```python
from build123d import *

# Parameters (mm, degrees)
F0_R     = 15
F0_R_2   = 10
F1_DEPTH = 25
F2_DEPTH = 50
F3_R     = 3


with BuildPart() as f1:
    # F0 (on Front) → F1 (new body)
    with BuildSketch(Plane.XZ):
        with BuildLine():
            ThreePointArc((-6.25, -29.341736), (18.874586, -23.318448), (30, 0))
            ThreePointArc((30, 0), (18.874586, 23.318448), (-6.25, 29.341736))
            ThreePointArc((-6.25, 29.341736), (-30, 0), (-6.25, -29.341736))
        make_face()
        Circle(F0_R, mode=Mode.SUBTRACT)
        with BuildLine():
            ThreePointArc((-6.25, -29.341736), (-30, 0), (-6.25, 29.341736))
            Line((-6.25, 29.341736), (-63.645833, 17.116013))
            ThreePointArc((-63.645833, 17.116013), (-48.989825, 13.602428), (-42.5, 0))
            ThreePointArc((-42.5, 0), (-48.989825, -13.602428), (-63.645833, -17.116013))
            Line((-63.645833, -17.116013), (-6.25, -29.341736))
        make_face()
        with BuildLine():
            ThreePointArc((-42.5, 0), (-48.989825, 13.602428), (-63.645833, 17.116013))
            ThreePointArc((-63.645833, 17.116013), (-77.5, 0), (-63.645833, -17.116013))
            ThreePointArc((-63.645833, -17.116013), (-48.989825, -13.602428), (-42.5, 0))
        make_face()
        with Locations((-60, 0)):
            Circle(F0_R_2, mode=Mode.SUBTRACT)
    extrude(amount=F1_DEPTH)

    # F0 (on Front) → F2 (join)
    with BuildSketch(Plane.XZ):
        with BuildLine():
            ThreePointArc((-6.25, -29.341736), (18.874586, -23.318448), (30, 0))
            ThreePointArc((30, 0), (18.874586, 23.318448), (-6.25, 29.341736))
            ThreePointArc((-6.25, 29.341736), (-30, 0), (-6.25, -29.341736))
        make_face()
        Circle(F0_R, mode=Mode.SUBTRACT)
    extrude(amount=F2_DEPTH)

    # F3
    f3_edges = [f1.edges().sort_by_distance(p)[0] for p in [
        (6.25, -50, -29.341736),
        (30, 0, 0),
        (-34.947917, 0, -23.228875),
        (-77.5, 0, 0),
        (-34.947917, 0, 23.228875),
    ]]
    fillet(f3_edges, radius=F3_R)


solid = f1.part
```
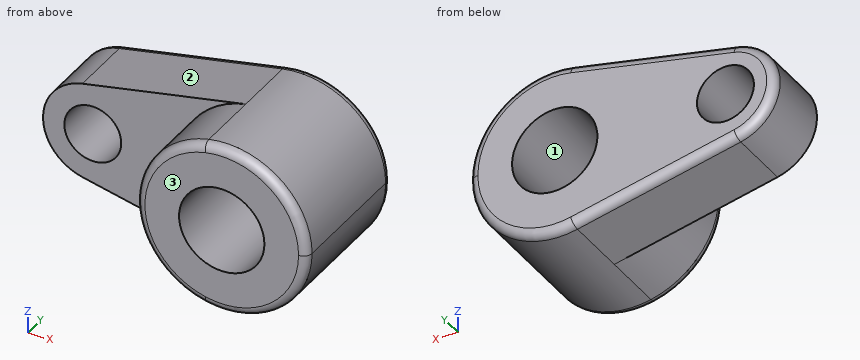
Can you work these out from the model? Positions are in its coordinate system, mm. Face numbers are marked on the shaded views. Coordinates: 2 decimals unless noted, no trailing zeros. Order: outer loops, then holes, each group sorted by start corner. A loop starts at its lowest first (then second) coordinate and runs counter-clockwise, first axis right, second up.
1. I need wall thicknesses on line 1 (Z direction, x = 0, y = -27); line 2 (X direction, y = -6, z = -2.5); line 3 (X direction, y = -16, z = -6). Which ranges of each line are inside material? Lowest first, please.
2. If we section it at B-B (y = -31): Please give me the cut outline in (x, z), then the cut area to 3 significant figures.
3. If we section it at A-A (y = -8.5): Please give me the cut outline in (x, z), then the cut area to 3 significant figures.
4. Thinking about a two-plate mould opening in Z: for the marked faces 1, 2 and 3, which applies, +Z half, -Z half, draft (parallel to the pull), parting line (faces both ways), or undercut?
5. I'm going to push flat-ended pins straight in: pin 1 (2 mm diameter, centred on x = -62.5, y = -15, fed in from -Z); pin 2 (12 mm diameter, centred on x = -60, z = 0, fed in from -Y); pin 3 (8 mm diameter, centred on y = -22, z = -13, fed in from +X); pin 4 (4 mm diameter, centred on x = -12.5, y = -10.5, fed in from -Z). Where does each tip first touch, or does it pass through?
Entries:
1. line 1: z = -30 to -15, 15 to 30
1. line 2: x = -77.32 to -69.68, -50.32 to -14.79, 14.79 to 29.9
1. line 3: x = -76.44 to -68, -52 to -13.75, 13.75 to 29.39
2. outline: (-6.25, -29.34) arc R30 ccw to (30, 0) arc R30 ccw to (-6.25, 29.34) arc R30 ccw to start; hole circle Ø30 at (0, 0)
2. area: 2,120 mm2
3. outline: (-63.65, -17.12) - (-6.25, -29.34) arc R30 ccw to (30, 0) arc R30 ccw to (-6.25, 29.34) - (-63.65, 17.12) arc R17.5 ccw to start; hole circle Ø20 at (-60, 0); hole circle Ø30 at (0, 0)
3. area: 3,790 mm2
4. face 1: undercut
4. face 2: +Z half
4. face 3: draft
5. pin 1: stops at z = -17.57
5. pin 2: passes through
5. pin 3: stops at x = 28.62
5. pin 4: stops at z = -28.44
